from build123d import *

# Parameters (mm, degrees)
F1_DEPTH = 5


with BuildPart() as f1:
    # F0 (on Top) → F1 (new body)
    with BuildSketch(Plane.XY):
        with BuildLine():
            ThreePointArc((3.0449996355, -0.1745772603), (3.0487496526, -0.0873244288), (3.05, 0))
            ThreePointArc((3.05, 0), (3.0487496526, 0.0873244288), (3.0449996355, 0.1745772603))
            ThreePointArc((3.0449996355, 0.1745772603), (1.6011501733, 0.55771632), (0.140706095, 0.2437101054))
            ThreePointArc((0.140706095, 0.2437101054), (0.1476756796, 0.1219436265), (0.15, 0))
            ThreePointArc((0.15, 0), (0.1476756796, -0.1219436265), (0.140706095, -0.2437101054))
            ThreePointArc((0.140706095, -0.2437101054), (1.6011501733, -0.55771632), (3.0449996355, -0.1745772603))
        make_face()
        with BuildLine():
            ThreePointArc((0.140706095, 0.2437101054), (-0.3175785854, 1.6654948853), (-1.3713114754, 2.724335669))
            ThreePointArc((-1.3713114754, 2.724335669), (-1.525, 2.6413774815), (-1.6736881601, 2.5497584087))
            ThreePointArc((-1.6736881601, 2.5497584087), (-1.2835715879, 1.1077785653), (-0.28141219, 0))
            ThreePointArc((-0.28141219, 0), (-0.075, 0.1299038106), (0.140706095, 0.2437101054))
        make_face()
        with BuildLine():
            ThreePointArc((0.15, 0), (0.1476756796, 0.1219436265), (0.140706095, 0.2437101054))
            ThreePointArc((0.140706095, 0.2437101054), (-0.075, 0.1299038106), (-0.28141219, 0))
            ThreePointArc((-0.28141219, 0), (-0.075, -0.1299038106), (0.140706095, -0.2437101054))
            ThreePointArc((0.140706095, -0.2437101054), (0.1476756796, -0.1219436265), (0.15, 0))
        make_face()
        with BuildLine():
            ThreePointArc((-1.6736881601, -2.5497584087), (-1.525, -2.6413774815), (-1.3713114754, -2.724335669))
            ThreePointArc((-1.3713114754, -2.724335669), (-0.3175785854, -1.6654948853), (0.140706095, -0.2437101054))
            ThreePointArc((0.140706095, -0.2437101054), (-0.075, -0.1299038106), (-0.28141219, 0))
            ThreePointArc((-0.28141219, 0), (-1.2835715879, -1.1077785653), (-1.6736881601, -2.5497584087))
        make_face()
    extrude(amount=F1_DEPTH)


solid = f1.part
Could you check a few things on this model? Use its own coordinates, in mm. Give positions to 0.01 mm unless a question says otherwise; leave off trailing zeros. Order: outer loops, then holes, each group sorted by start corner. A loop starts at its lowest first (then second) coordinate and runs counter-clockwise, first axis right, second up.
Item 1: If we section it at B-B, the plane x = 1.45: Write out the boundary of the cut face in (y, z).
Item 2: If we section it at A-A, the plane z = 3.35: Write out the boundary of the cut face in (x, y) (3 decimals), plus the area to 3 significant figures.
Item 3: If we section it at C-C, the plane y = 1.7: Write out the boundary of the cut face in (x, z), plus the area to 3 significant figures.
Item 4: If we mould it in two halves opening along Y, with no side actions, what happens to faces 1 (the face through (-1.273, -1.089, 2.465)), 2 (the face through (0, 0, 0))? For each: pulls with the +Y half, pulls with the -Y half, needs draft (parallel to the pull), parting line crosses it, or undercut.
Item 5: I need wall thicknesses on line 1 (Y direction, x = -1.35, z = 0.8); line 2 (Y direction, x = 1.5, z = 2); line 3 (Y direction, x = 2.75, z = 4.55). Which ranges of each line are inside material? Lowest first, please.
Values:
1. outline: (-0.56, 0) - (0.56, 0) - (0.56, 5) - (-0.56, 5) - close
2. outline: (-1.674, -2.55) arc R3.05 ccw to (-1.371, -2.724) arc R3.2 ccw to (0.141, -0.244) arc R3.2 ccw to (3.045, -0.175) arc R3.05 ccw to (3.045, 0.175) arc R3.2 ccw to (0.141, 0.244) arc R3.2 ccw to (-1.371, 2.724) arc R3.05 ccw to (-1.674, 2.55) arc R3.2 ccw to (-0.281, 0) arc R3.2 ccw to start
2. area: 7.85 mm2
3. outline: (-1.53, 0) - (-0.34, 0) - (-0.34, 5) - (-1.53, 5) - close
3. area: 5.97 mm2
4. face 1: undercut
4. face 2: needs draft
5. line 1: y = -2.71 to -1.24, 1.24 to 2.71
5. line 2: y = -0.56 to 0.56
5. line 3: y = -0.31 to 0.31
